```python
from build123d import *


with BuildPart() as part:
    # Sketch1 → Revolve1 (revolve)
    with BuildSketch(Plane(origin=(0, 0, 0), x_dir=(-1, 0, 0), z_dir=(0, 0, -1))):
        with BuildLine():
            Line((-22.4, 5.033333333), (-22.5, 5.033333333))
            Line((-22.5, 5.033333333), (-22.5, 4))
            Line((-22.5, 4), (22.5, 4))
            Line((22.5, 4), (22.5, 5.033333333))
            Line((22.5, 5.033333333), (22.4, 5.033333333))
            Line((22.4, 5.033333333), (22.4, 5.133333333))
            Line((22.4, 5.133333333), (22.5, 5.133333333))
            Line((22.5, 5.133333333), (22.5, 6.3))
            ThreePointArc((22.5, 6.3), (22.441421356, 6.441421356), (22.3, 6.5))
            Line((22.3, 6.5), (17.55, 6.5))
            Line((17.55, 6.5), (17.55, 6.2))
            Line((17.55, 6.2), (16.4, 6.2))
            Line((16.4, 6.2), (16.4, 6.5))
            Line((16.4, 6.5), (-16.4, 6.5))
            Line((-16.4, 6.5), (-16.4, 6.2))
            Line((-16.4, 6.2), (-17.55, 6.2))
            Line((-17.55, 6.2), (-17.55, 6.5))
            Line((-17.55, 6.5), (-22.3, 6.5))
            ThreePointArc((-22.3, 6.5), (-22.441421356, 6.441421356), (-22.5, 6.3))
            Line((-22.5, 6.3), (-22.5, 5.133333333))
            Line((-22.5, 5.133333333), (-22.4, 5.133333333))
            Line((-22.4, 5.133333333), (-22.4, 5.033333333))
        make_face()
    revolve(axis=Axis((22.5, 0, 0), (-1, 0, 0)))


solid = part.part
```
Check sheet for the modelled part. Datum: model origin and axes. Units: mm. Round coordinates to 2 decimals unless told otherwise and drop trailing zeros. Loops run counter-clockwise (first coordinate to the right, second up) from the corner with the lowest first, then second, coordinate; pieces in that order, holes last. Notation, with made-up numbers: (-32, 84.5) -> (20, 84.5) arc R27 ccw to (20, 109.5) -> close; hole circle Ø8 at (59, 14.5). An arc over 180 degrees is marked (long way). Answer in a Markdown table with one row per item.
Q1. Release check for a two-part mould opening along X. For faces 1 (the face through (-16.97, 2.86, 5.5)), 2 (the face through (0.23, -5.158, 3.955)), 3 (the face through (22.5, -2, 5)), 4 (the face through (-22.5, 2, -4)) record: released by +X, released by -X, zero draft, split by the parting line, or undercut.
Data:
| item | result |
|---|---|
| face 1 | undercut |
| face 2 | zero draft |
| face 3 | released by +X |
| face 4 | released by -X |
Q2. Thickness scan on L1, parallel to X at y = -5.5, z = 3; L2, parallel to Y at x = -5.5, z = 0. Record the ranges inside material, lowest first.
Data:
| item | result |
|---|---|
| L1 | x = -22.5 to -17.55, -16.4 to 16.4, 17.55 to 22.5 |
| L2 | y = -6.5 to -4, 4 to 6.5 |
Q3. Sectioned sample at A-A on x = -13.5. Enter the section's corners in (y, z), then the cut area to 3 significant figures.
Data:
| item | result |
|---|---|
| outline | circle Ø13 at (0, 0); hole circle Ø8 at (0, 0) |
| area | 82.5 mm^2 |
Q4. Go/stop test with flat-tipped pins: P1, Ø3, axis at x = 7, z = 5, coming from the -Y side; P2, Ø6, axis at y = 0, z = 0, coming from the +X side; P3, Ø6, axis at x = 5, z = -5, coming from the -Y side; P4, Ø3, axis at x = 11, y = 3, coming from the +Z side. Record where each tip stops, or that it passes through.
Data:
| item | result |
|---|---|
| P1 | stops at y = -5.48 |
| P2 | passes through |
| P3 | stops at y = -6.18 |
| P4 | stops at z = 6.32 |
